Input: part model. Units: mm. Frame: model coordinates. A direction names the side the tool comes from. Round coordinates to 2 decimals unless told otherwise and drop trailing zeros. Write each loop counter-clockwise with the first axis right and the second up, starting at its lowest first coordinate (ties: lowest second). Pieces come first, ordered by that corner, then holes. Notation, with made-up numbers: (75, 2.25) - (89, 2.25) arc R30 ccw to (89, 27.25) - close; hole circle Ø7 at (52.5, -9). An arc over 180 degrees is marked (long way). One line per item, written item: value. Start each with the question number.
```python
from build123d import *

# Parameters (mm, degrees)
SKETCH1_W           = 15
SKETCH1_H           = 40
SKETCH1_R           = 1.5
BOSS_EXTRUDE2_DEPTH = 1
BOSS_EXTRUDE5_START = -8
BOSS_EXTRUDE5_DEPTH = 8
LPATTERN2_COUNT     = 2
LPATTERN2_PITCH     = 16
SKETCH6_R           = 0.75
CUT_EXTRUDE3_DEPTH  = 40


with BuildPart() as part:
    # Sketch1 → Boss-Extrude2 (new body)
    with BuildSketch(Plane.XY):
        Rectangle(SKETCH1_W, SKETCH1_H)
        with Locations((0, 12)):
            Circle(SKETCH1_R, mode=Mode.SUBTRACT)
        with Locations((0, -12)):
            Circle(SKETCH1_R, mode=Mode.SUBTRACT)
    extrude(amount=BOSS_EXTRUDE2_DEPTH)

    # Sketch5 → Boss-Extrude5 (add)
    with BuildSketch(Plane(origin=(0, 20, 0), x_dir=(1, 0, 0), z_dir=(0, 1, 0)).offset(BOSS_EXTRUDE5_START)):
        with BuildLine():
            Line((7.5, -0.5), (7.5, -1))
            ThreePointArc((7.5, -1), (8.383883476, -0.633883476), (8.75, 0.25))
            ThreePointArc((8.75, 0.25), (7.374363797, 1.493670191), (6.275255129, 0))
            Line((6.275255129, 0), (6.792893219, 0))
            ThreePointArc((6.792893219, 0), (7.373173516, 0.98919892), (8.25, 0.25))
            ThreePointArc((8.25, 0.25), (8.030330086, -0.280330086), (7.5, -0.5))
        make_face()
        with BuildLine():
            ThreePointArc((6.275255129, 0), (6.709430585, -0.718245837), (7.5, -1))
            Line((7.5, -1), (7.5, -0.5))
            ThreePointArc((7.5, -0.5), (7.066987298, -0.362372436), (6.792893219, 0))
            Line((6.792893219, 0), (6.275255129, 0))
        make_face()
    boss_extrude5 = extrude(amount=-BOSS_EXTRUDE5_DEPTH)

    # LPattern2: Boss-Extrude5 ×2
    with Locations(*[(0, -i * LPATTERN2_PITCH, 0) for i in range(1, LPATTERN2_COUNT)]):
        add(boss_extrude5)

    # Sketch6 → Cut-Extrude3 (cut)
    with BuildSketch(Plane(origin=(0, 20, 0), x_dir=(1, 0, 0), z_dir=(0, 1, 0))):
        with Locations((7.5, 0.25)):
            Circle(SKETCH6_R)
    extrude(amount=-CUT_EXTRUDE3_DEPTH, mode=Mode.SUBTRACT)


solid = part.part
```
Q1. Material intervals for probe 1 along Y at (x, z) = (0, 0.6); probe 2 along Z at (x, y) = (7.5, 9); probe 3 along X at (y, z) = (9, -0.2), sorted ascending. Write a range as from..to.
Q2. Cut plane B-B, the plane y = -13. Output: boundary loops of the cut face in (x, z).
Q3. Pull-direction query (X, two-part tool) for faces 1 (the flat face through (-0.1, 20, 0.5)), 2 (the flat face through (-7.5, -0.3, 0.5)), 3 (the cylindrical face through (-0.325, -13.464, 0.493)); classes: pulls with the +X half, pulls with the -X half, needs draft (parallel to the pull), parting line crosses it, or undercut.
Q4. Access query for faces 4 (the flat face through (8, -4, -1)), 5 (the flat face through (8, 12, -1)), 6 (the flat face through (8, -12, -1)). Directions: +Z, -Z, +X, -X, +Y, -Y. A direction counts if a zero-diameter tool reaches every point of the face in a straight line with its end or side. Return the directions, or none.
Q5. Cut plane C-C, the plane y = -3. Output: boundary loops of the cut face in (x, z), and give its area (3 significant figures).
Q6. Contact query for flat-ended pins moving along their axis: pin 1 Ø5 at (x, y) = (-6, -9) entering from -Z; pin 2 Ø2.5 at (x, y) = (0, -12) entering from -Z; pin 3 Ø0.7 at (x, z) = (8, 0) entering from +Y. Output: stop coordinate, or through.
Q7. Cut plane D-D, the plane x = 5.75. Output: boundary loops of the cut face in (y, z).
Q8. Cut plane A-A, the plane x = 0. Output: boundary loops of the cut face in (y, z).
A:
1. probe 1: y = -20..-13.5, -10.5..10.5, 13.5..20
1. probe 2: z = -1.5..-1, 0.5..1
1. probe 3: x = 6.25..6.75, 8.25..8.75
2. outline: (-7.5, 0) - (-1.12, 0) - (-1.12, 1) - (-7.5, 1) - close; (1.12, 0) - (6.79, 0) arc R0.75 cw to (7.5, 0.5) - (7.5, 1) - (1.12, 1) - close
3. face 1: needs draft
3. face 2: pulls with the -X half
3. face 3: undercut
4. face 4: -Z, +X
4. face 5: -Z, +X, +Y
4. face 6: -Z, +X, -Y
5. outline: (-7.5, 0) - (6.79, 0) arc R0.75 cw to (7.5, 0.5) - (7.5, 1) - (-7.5, 1) - close
5. area: 14.7 mm²
6. pin 1: stops at z = 0
6. pin 2: passes through
6. pin 3: stops at y = 12
7. outline: (-20, 0) - (20, 0) - (20, 1) - (-20, 1) - close
8. outline: (-20, 0) - (-13.5, 0) - (-13.5, 1) - (-20, 1) - close; (-10.5, 0) - (10.5, 0) - (10.5, 1) - (-10.5, 1) - close; (13.5, 0) - (20, 0) - (20, 1) - (13.5, 1) - close
